Autodesk Inventor part; units mm, degrees
ref_plane "YZ Plane" through (0, 0, 0) normal (1, 0, 0) x (0, 1, 0)
ref_plane "XZ Plane" through (0, 0, 0) normal (0, 1, 0) x (-1, 0, 0)
ref_plane "XY Plane" through (0, 0, 0) normal (0, 0, 1) x (1, 0, 0)
sketch "Sketch1" plane through (0, 0, 0) normal (0, 1, 0) x (-1, 0, 0)
  line L0 (0, 0) -> (0, -1219.2)
  line L1 (0, 0) -> (88.9, 0)
  line L2 (88.9, 0) -> (88.9, -1219.2)
  line L3 (88.9, -1219.2) -> (0, -1219.2)
  line L4 (0, 0) -> (0, 1219.2) construction
  line L5 (0, 1219.2) -> (1219.2, 1219.2) construction
  line L6 (0, 1219.2) -> (0, 3657.6) construction
  line L7 (0, 3657.6) -> (0, 4876.8) construction
  line L8 (0, 4876.8) -> (0, 6096) construction
  line L9 (0, -1219.2) -> (2438.4, -1219.2) construction
  line L10 (0, 6096) -> (2438.4, 6096) construction
  line L11 (2438.4, 6096) -> (2438.4, -1219.2) construction
  line L12 (0, 3657.6) -> (0, 3352.8) construction
  line L13 (0, 3352.8) -> (2438.4, 3352.8) construction
  line L14 (2438.4, 3352.8) -> (1219.2, 3352.8)
  line L15 (1219.2, 3352.8) -> (1219.2, 3263.9)
  line L16 (1219.2, 3263.9) -> (2438.4, 3263.9)
  line L17 (2438.4, 3263.9) -> (2438.4, 3352.8)
  line L18 (0, 6096) -> (862.1046, 6958.1046)
  line L19 (862.1046, 6958.1046) -> (924.9664, 6895.2428)
  line L20 (924.9664, 6895.2428) -> (62.8618, 6033.1382)
  line L21 (62.8618, 6033.1382) -> (0, 6096)
  line L22 (0, 4876.8) -> (1219.2, 4876.8) construction
  line L23 (1219.2, 4876.8) -> (2081.3046, 5738.9046)
  line L24 (1219.2, 1219.2) -> (2081.3046, 357.0954)
  line L25 (2081.3046, 357.0954) -> (2018.4428, 294.2336)
  line L26 (2018.4428, 294.2336) -> (1156.3382, 1156.3382)
  line L27 (1156.3382, 1156.3382) -> (1219.2, 1219.2)
  line L28 (2018.4428, 294.2336) -> (88.9, -1219.2)
  line L29 (2081.3046, 357.0954) -> (2144.1664, 419.9572)
  line L30 (2144.1664, 419.9572) -> (1282.0618, 1282.0618)
  line L31 (1282.0618, 1282.0618) -> (1219.2, 1219.2)
  line L32 (2438.4, 3352.8) -> (2438.4, 3441.7)
  line L33 (2438.4, 3441.7) -> (1219.2, 3441.7)
  line L34 (1219.2, 3441.7) -> (1219.2, 3352.8)
  line L35 (1156.3382, 4939.6618) -> (1282.0618, 4813.9382)
  line L36 (2018.4428, 5801.7664) -> (2144.1664, 5676.0428)
  line L37 (1282.0618, 4813.9382) -> (2144.1664, 5676.0428)
  line L38 (2018.4428, 5801.7664) -> (1156.3382, 4939.6618)
  line L39 (2018.4428, 5801.7664) -> (924.9664, 6895.2428)
  line L40 (62.8618, 6033.1382) -> (1156.3382, 4939.6618)
  line L41 (1233.6206, 4168.8855) -> (1267.6412, 4086.7527)
  line L42 (1263.7078, 2313.9849) -> (1230.0006, 2231.7229)
  arc A0 (862.1046, 6958.1046) -> (0, 6096) centre (431.0523, 6527.0523) ccw
  line L43 (1246.8542, 2272.8539) -> (2375.0183, 1810.583)
  line L44 (2391.8719, 1851.7139) -> (2358.1646, 1769.452)
  line L45 (2391.8719, 1851.7139) -> (1263.7078, 2313.9849)
  line L46 (1230.0006, 2231.7229) -> (2358.1646, 1769.452)
  line L47 (1230.0006, 2231.7229) -> (1219.2, 3263.9)
  line L48 (2144.1664, 419.9572) -> (2391.8719, 1851.7139)
  line L49 (2391.8719, 1851.7139) -> (2438.4, 3263.9)
  line L50 (1219.2, 3441.7) -> (1233.6206, 4168.8855)
  line L51 (1250.6309, 4127.8191) -> (2377.0248, 4594.3867)
  line L52 (2360.0145, 4635.4532) -> (2394.0351, 4553.3203)
  line L53 (2394.0351, 4553.3203) -> (1267.6412, 4086.7527)
  line L54 (2360.0145, 4635.4532) -> (1233.6206, 4168.8855)
  line L55 (2394.0351, 4553.3203) -> (2144.1664, 5676.0428)
  line L56 (2438.4, 3441.7) -> (2394.0351, 4553.3203)
  line L57 (2144.1664, 5676.0428) -> (2057.3895, 5656.7301)
  line L58 (2394.0351, 4553.3203) -> (2305.2058, 4549.7751)
  line L59 (2394.0351, 4553.3203) -> (2307.2582, 4534.0076)
  line L60 (2307.2582, 4534.0076) -> (2057.3895, 5656.7301)
  line L61 (2438.4, 3441.7) -> (2349.5707, 3438.1548)
  line L62 (2349.5707, 3438.1548) -> (2305.2058, 4549.7751)
  line L63 (1219.2, 3441.7) -> (1308.0825, 3439.9374)
  line L64 (1233.6206, 4168.8855) -> (1322.5031, 4167.1229)
  line L65 (1322.5031, 4167.1229) -> (1308.0825, 3439.9374)
  line L66 (2018.4428, 5801.7664) -> (1955.581, 5738.9046)
  line L67 (1955.581, 5738.9046) -> (862.1046, 6832.381)
  line L68 (924.9664, 6895.2428) -> (862.1046, 6832.381)
  line L69 (62.8618, 6033.1382) -> (125.7236, 6096)
  line L70 (62.8618, 6033.1382) -> (125.7236, 6096)
  line L71 (125.7236, 6096) -> (1219.2, 5002.5236)
  line L72 (1156.3382, 1156.3382) -> (0, 0)
  line L73 (0, 0) -> (62.8618, -62.8618)
  line L74 (1156.3382, 1156.3382) -> (1219.2, 1093.4764)
  line L75 (1219.2, 1093.4764) -> (62.8618, -62.8618)
  line L76 (2018.4428, 294.2336) -> (1963.5776, 364.1837)
  line L77 (88.9, -1219.2) -> (34.0348, -1149.2499)
  line L78 (34.0348, -1149.2499) -> (1963.5776, 364.1837)
  line L79 (2144.1664, 419.9572) -> (2056.5677, 435.1125)
  line L80 (2391.8719, 1851.7139) -> (2304.2732, 1866.8692)
  line L81 (2391.8719, 1851.7139) -> (2303.0201, 1854.6414)
  line L82 (2304.2732, 1866.8692) -> (2056.5677, 435.1125)
  line L83 (1230.0006, 2231.7229) -> (1318.8957, 2232.6531)
  line L84 (1219.2, 3263.9) -> (1308.0951, 3264.8302)
  line L85 (1308.0951, 3264.8302) -> (1318.8957, 2232.6531)
  line L86 (2438.4, 3263.9) -> (2349.5482, 3266.8275)
  line L87 (2349.5482, 3266.8275) -> (2303.0201, 1854.6414)
  line L88 (88.9, 0) -> (125.7236, 0)
  line L89 (1233.6206, 4168.8855) -> (1219.2, 4876.8)
  line L90 (1233.6206, 4168.8855) -> (1322.5022, 4170.6961)
  line L91 (1219.2, 4876.8) -> (1308.0816, 4878.6106)
  line L92 (1308.0816, 4878.6106) -> (1322.5022, 4170.6961)
  line L93 (1282.0618, 4813.9382) -> (1309.9674, 4786.0326)
  line L94 (1267.6412, 4086.7527) -> (1318.4756, 3964.0275)
  line L95 (2360.0145, 4635.4532) -> (2374.4273, 4641.4231)
  line L96 (1230.0006, 2231.7229) -> (1219.2, 1219.2)
  line L97 (1230.0006, 2231.7229) -> (1318.8955, 2230.7747)
  line L98 (1219.2, 1219.2) -> (1308.0949, 1218.2518)
  line L99 (1308.0949, 1218.2518) -> (1318.8955, 2230.7747)
  line L100 (1282.0618, 1282.0618) -> (1309.0636, 1309.0636)
  line L101 (1263.7078, 2313.9849) -> (1316.7428, 2438.4)
  line L102 (2358.1646, 1769.452) -> (2376.5379, 1763.082)
  point P0 (1770.957, 2057.4547)
  point P1 (1955.1236, 357.5528)
  point P2 (88.9, -1106.2164)
  point P3 (2292.1025, 1796.5213)
  point P4 (2067.2525, 496.8711)
  dimension "d0" = 1219.2
  dimension "d2" = 1219.2
  dimension "d3" = 1219.2
  dimension "d16" = 2438.4
  dimension "d17" = 1219.2
  dimension "d18" = 1219.2
  dimension "d20" = 2438.4
  dimension "d21" = 304.8
  dimension "d22" = 1219.2
  dimension "d23" = 88.9
  dimension "d24" = 1219.2
  dimension "d25" = 45
  dimension "d26" = 88.9
  dimension "d27" = 1219.2
  dimension "d28" = 1219.2
  dimension "d29" = 1219.2
  dimension "d31" = 1219.2
  dimension "d32" = 88.9
  dimension "d33" = 88.9
  dimension "d34" = 88.9
  dimension "d35" = 177.8
  dimension "d36" = 177.8
  dimension "d38" = 88.9
  dimension "d39" = 88.9
  dimension "d43" = 1219.2
  dimension "d44" = 88.9
  dimension "d45" = 1219.2
  dimension "d46" = 88.9
  dimension "d47" = 88.9
  dimension "d48" = 88.9
  dimension "d49" = 88.9
  dimension "d50" = 88.9
  dimension "d51" = 88.9
  dimension "d54" = 88.9
  dimension "d55" = 88.9
  dimension "d57" = 88.9
  dimension "d58" = 88.9
  dimension "d59" = 88.9
  dimension "d60" = 88.9
  dimension "d61" = 88.9
  dimension "d64" = 88.9
  dimension "d65" = 88.9
  dimension "d66" = 88.9
  dimension "d69" = 88.9
  dimension "d70" = 88.9
  dimension "d71" = 88.9
  dimension "d72" = 88.9
extrude "Extrusion1" add sketch "Sketch1" along normal blind 38.1 contours L30 L82 L46 L102 L48 | L102 L44 L48
properties part number "S_2x4x57.206"
Verification items for the finished model (mm, model axes). A direction names the side the tool comes from. Give positions to 0.01 mm unless a question says otherwise; leave off trailing zeros. Order: outer loops, then holes, each group sorted by start corner. A loop starts at its lowest first (then second) coordinate and runs counter-clockwise, first axis right, second up. Notation, with made-up numbers: M -40,27.25 L 2,27.25 A17 cw 2,59.25 Z; hole C -1,-32 d10. An arc over 180 degrees is marked long. Answer as a JSON object with one key per item and string values. Group by question number.
1) Scan lines: line 1 along X through (y, z) = (18, 1794); line 2 along X through (y, z) = (36, 1029.5); line 3 along X through (y, z) = (20.5, 631.5). Record each from-to range of solid material in increasing order. Write a range as [from, to].
2) Cross-section at A-A (y = 7). Enter the section's corners in (x, z).
3) Cross-section at C-C (z = 948.5). Enter the section's corners in (x, y).
4) Cross-section at B-B (x = -2227). Enter the section's corners in (y, z).
5) Access from +Z, -Z, +X, -X, +Y, -Y to the whole of each face (thin tool, end or side, straight path). Record for faces 1 (the face through (-2375.254, 18.783, 1811.159)), 2 (the face through (-2217, 0, 1139)).
6) Depth check by flat-ended pin: pin 1 Ø1.5 at (y, z) = (22, 988) entering from -X; pin 2 Ø2 at (y, z) = (32, 1546.5) entering from -X; pin 3 Ø12 at (x, y) = (-2148, 13) entering from -Z. Enter the tip coordinate at first touch or a pass-through.
7) Mould release check, pull along X, two halves, no side actions. Record for faces 3 (the face through (-2324.671, 18.783, 1783.176)), 4 (the face through (-2217, 38.1, 1139)), 5 (the face through (-2181.25, 18.78, 1155.79)): released by +X, released by -X, zero draft, split by the parting line, or undercut.
Result sheet:
{
 "1": {"line 1": "x = [-2381.89, -2368.22], [-2298.26, -2291.67]", "line 2": "x = [-2249.62, -2159.4]", "line 3": "x = [-2180.77, -2090.54]"},
 "2": {"outline": "M -2391.87,1851.71 L -2144.17,419.96 L -2067.25,496.87 L -2292.1,1796.52 L -2358.16,1769.45 Z"},
 "3": {"outline": "M -2235.61,0 L -2145.39,0 L -2145.39,38.1 L -2235.61,38.1 Z"},
 "4": {"outline": "M 0,898.74 L 38.1,898.74 L 38.1,1420.22 L 0,1420.22 Z"},
 "5": {"face 1": "+Z, +Y, -Y", "face 2": "+Z, -Z, +X, -X, -Y"},
 "6": {"pin 1": "stops at x = -2242.57", "pin 2": "stops at x = -2339.24", "pin 3": "stops at z = 419.96"},
 "7": {"face 3": "undercut", "face 4": "zero draft", "face 5": "released by +X"}
}
